Geometry: final body of the model. Coordinates: model frame, mm. Face numbers are marked on the shaded views. A direction names the side the tool comes from. Give positions to 0.01 mm unless a question says otherwise; leave off trailing zeros. Loops run counter-clockwise (first coordinate to the right, second up) from the corner with the lowest first, then second, coordinate; pieces in that order, holes last.
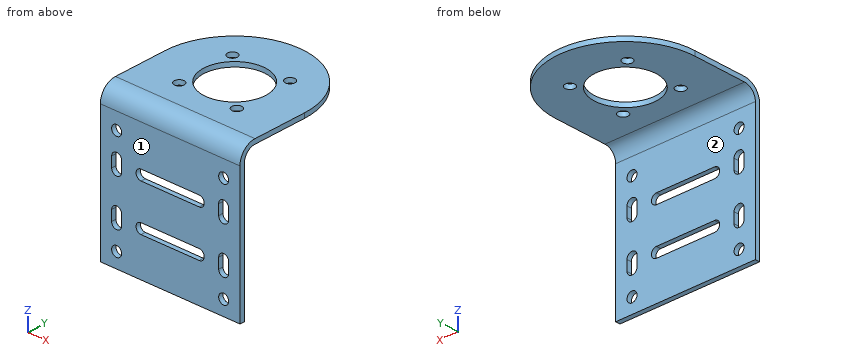
from build123d import *

# Parameters (mm, degrees)
BOSS_EXTRUDE2_DEPTH          = 2
SKETCH2_R                    = 13.25
CUT_EXTRUDE1_DEPTH           = 62.54645277
EDGE_FLANGE1_STRIP_W         = 18
EDGE_FLANGE1_STRIP_H         = 2
EDGE_FLANGE1_STRIP_CUT_DEPTH = 60
EDGE_FLANGE1_DEPTH           = 60
SKETCH12_R                   = 2.1
CUT_EXTRUDE2_DEPTH           = 89.718717014
SKETCH13_R                   = 2.15
CUT_EXTRUDE3_DEPTH           = 2


# Sheet-metal steps are written as plain solids
with BuildPart() as part:
    # Sketch1 → Boss-Extrude2 (new body)
    with BuildSketch(Plane.XY):
        with BuildLine():
            Line((51.588785047, -26.495327103), (-8.411214953, -26.495327103))
            Line((-8.411214953, -26.495327103), (-8.411214953, 3.504672897))
            ThreePointArc((-8.411214953, 3.504672897), (21.588785047, 33.504672897), (51.588785047, 3.504672897))
            Line((51.588785047, 3.504672897), (51.588785047, -26.495327103))
        make_face()
    extrude(amount=BOSS_EXTRUDE2_DEPTH)

    # Sketch2 → Cut-Extrude1 (cut, through all)
    with BuildSketch(Plane.XY.offset(2)):
        with Locations((21.588785047, 3.504672897)):
            Circle(SKETCH2_R)
    extrude(amount=-CUT_EXTRUDE1_DEPTH, mode=Mode.SUBTRACT)

    # Edge-Flange1 strip (across the edge) → Edge-Flange1 strip cut (cut)
    with BuildSketch(Plane(origin=(51.588785047, -26.495327103, 0), x_dir=(0, 1, 0), z_dir=(-1, 0, 0))):
        with Locations((-2, -1)):
            Rectangle(EDGE_FLANGE1_STRIP_W, EDGE_FLANGE1_STRIP_H)
    extrude(amount=EDGE_FLANGE1_STRIP_CUT_DEPTH, mode=Mode.SUBTRACT)

    # Edge-Flange1 section (across the edge) → Edge-Flange1 (add)
    with BuildSketch(Plane(origin=(51.588785047, -26.495327103, 0), x_dir=(0, 1, 0), z_dir=(-1, 0, 0))):
        with BuildLine():
            Line((0, 5), (0, 61.93))
            Line((0, 61.93), (2, 61.93))
            Line((2, 61.93), (2, 5))
            ThreePointArc((2, 5), (3.464466094, 1.464466094), (7, 0))
            Line((7, 0), (7, -2))
            ThreePointArc((7, -2), (2.050252532, 0.050252532), (0, 5))
        make_face()
    extrude(amount=EDGE_FLANGE1_DEPTH)

    # Sketch12 → Cut-Extrude2 (cut, through all)
    with BuildSketch(Plane.XY.offset(2)):
        with Locations((33.963153717, 15.879041568)):
            Circle(SKETCH12_R)
        with Locations((33.963153717, -8.869695774)):
            Circle(SKETCH12_R)
        with Locations((9.214416376, -8.869695774)):
            Circle(SKETCH12_R)
        with Locations((9.214416376, 15.879041568)):
            Circle(SKETCH12_R)
    extrude(amount=-CUT_EXTRUDE2_DEPTH, mode=Mode.SUBTRACT)

    # Sketch13 → Cut-Extrude3 (cut)
    with BuildSketch(Plane.XZ.offset(26.495327103)):
        with Locations(Location((-1.411214953, -12, 0), (0, 0, 270))):
            Circle(SKETCH13_R)
        with Locations(Location((44.588785047, -12, 0), (0, 0, 270))):
            Circle(SKETCH13_R)
        with Locations(Location((44.588785047, -55.6, 0), (0, 0, 270))):
            Circle(SKETCH13_R)
        with Locations(Location((-1.411214953, -55.6, 0), (0, 0, 270))):
            Circle(SKETCH13_R)
        with BuildLine():
            Line((-3.561214953, -41.3), (-3.561214953, -45.6))
            ThreePointArc((-3.561214953, -45.6), (-1.411214953, -47.75), (0.738785047, -45.6))
            Line((0.738785047, -45.6), (0.738785047, -41.3))
            ThreePointArc((0.738785047, -41.3), (-1.411214953, -39.15), (-3.561214953, -41.3))
        make_face()
        with BuildLine():
            Line((-3.561214953, -22), (-3.561214953, -26.3))
            ThreePointArc((-3.561214953, -26.3), (-1.411214953, -28.45), (0.738785047, -26.3))
            Line((0.738785047, -26.3), (0.738785047, -22))
            ThreePointArc((0.738785047, -22), (-1.411214953, -19.85), (-3.561214953, -22))
        make_face()
        with BuildLine():
            Line((46.738785047, -26.3), (46.738785047, -22))
            ThreePointArc((46.738785047, -22), (44.588785047, -19.85), (42.438785047, -22))
            Line((42.438785047, -22), (42.438785047, -26.3))
            ThreePointArc((42.438785047, -26.3), (44.588785047, -28.45), (46.738785047, -26.3))
        make_face()
        with BuildLine():
            Line((42.438785047, -41.3), (42.438785047, -45.6))
            ThreePointArc((42.438785047, -45.6), (44.588785047, -47.75), (46.738785047, -45.6))
            Line((46.738785047, -45.6), (46.738785047, -41.3))
            ThreePointArc((46.738785047, -41.3), (44.588785047, -39.15), (42.438785047, -41.3))
        make_face()
        with BuildLine():
            Line((9.088785047, -22), (34.088785047, -22))
            ThreePointArc((34.088785047, -22), (36.238785047, -24.15), (34.088785047, -26.3))
            Line((34.088785047, -26.3), (9.088785047, -26.3))
            ThreePointArc((9.088785047, -26.3), (6.938785047, -24.15), (9.088785047, -22))
        make_face()
        with BuildLine():
            Line((9.088785047, -41.3), (34.088785047, -41.3))
            ThreePointArc((34.088785047, -41.3), (36.238785047, -43.45), (34.088785047, -45.6))
            Line((34.088785047, -45.6), (9.088785047, -45.6))
            ThreePointArc((9.088785047, -45.6), (6.938785047, -43.45), (9.088785047, -41.3))
        make_face()
    extrude(amount=-CUT_EXTRUDE3_DEPTH, mode=Mode.SUBTRACT)


solid = part.part
Item 1: Section query D-D on z = -55.6. Return loops of the section in (x, y).
Values follow:
outline: (-8.41, -26.5) - (-3.56, -26.5) - (-3.56, -24.5) - (-8.41, -24.5) - close; (0.74, -26.5) - (42.44, -26.5) - (42.44, -24.5) - (0.74, -24.5) - close; (46.74, -26.5) - (51.59, -26.5) - (51.59, -24.5) - (46.74, -24.5) - close
Item 2: Pin query (flat end, axial travel): pin 1 (12 mm diameter, centred on x = -2.5, z = -45.5, fed in from +Y); pin 2 (5.5 mm diameter, centred on x = 9.21, y = 15.88, fed in from -Z); pin 3 (8 mm diameter, centred on x = 27.5, z = -25.5, fed in from -Y); pin 4 (1 mm diameter, centred on x = 17, y = -26, fed in from +Z). Return the tip coordinate at first contact, or that it passes through.
Values follow:
pin 1: stops at y = -24.5
pin 2: stops at z = 0
pin 3: stops at y = -26.5
pin 4: stops at z = -1.4
Item 3: Section query C-C on x = 20.5. Return loops of the section in (y, z), plus the area to 3 significant figures.
Values follow:
outline: (-26.5, -61.93) - (-24.5, -61.93) - (-24.5, -45.6) - (-26.5, -45.6) - close; (-26.5, -41.3) - (-24.5, -41.3) - (-24.5, -26.3) - (-26.5, -26.3) - close; (-26.5, -22) - (-24.5, -22) - (-24.5, -5) arc R5 cw to (-19.5, 0) - (-9.7, 0) - (-9.7, 2) - (-19.5, 2) arc R7 ccw to (-26.5, -5) - close; (16.71, 0) - (33.48, 0) - (33.48, 2) - (16.71, 2) - close
area: 169 mm2
Item 4: Set-up query: the marked faces 1 and 2. Return all of +Z, -Z, +X, -X, +Y, -Y with unobstructed straight access to the full face (end or side cutting, diameter ignored); none if empty.
Values follow:
face 1: +Z, -Z, +X, -X, -Y
face 2: -Z, +X, -X, +Y
Item 5: Section query A-A on z = -43.45. Return loops of the section in (x, y).
Values follow:
outline: (-8.41, -26.5) - (-3.56, -26.5) - (-3.56, -24.5) - (-8.41, -24.5) - close; (0.74, -26.5) - (6.94, -26.5) - (6.94, -24.5) - (0.74, -24.5) - close; (36.24, -26.5) - (42.44, -26.5) - (42.44, -24.5) - (36.24, -24.5) - close; (46.74, -26.5) - (51.59, -26.5) - (51.59, -24.5) - (46.74, -24.5) - close
Item 6: Ray query, probe 1 along X at (y, z) = (-25.35, -55.6); probe 2 along Z at (x, y) = (13, 28.5); probe 3 along Y at (x, z) = (10.5, -38). Return the intervals inside material, ascending.
Values follow:
probe 1: x = -8.41 to -3.56, 0.74 to 42.44, 46.74 to 51.59
probe 2: z = 0 to 2
probe 3: y = -26.5 to -24.5
Item 7: Section query B-B on y = 9.5. Return loops of the section in (x, z).
Values follow:
outline: (-7.81, 0) - (9.77, 0) - (9.77, 2) - (-7.81, 2) - close; (33.4, 0) - (50.98, 0) - (50.98, 2) - (33.4, 2) - close
